Could you check a few things on this model? Use its own coordinates, in mm. A direction names the side the tool comes from. Give positions to 0.01 mm unless a question says otherwise; leave off trailing zeros. Loops run counter-clockwise (first coordinate to the right, second up) from the corner with the lowest first, then second, coordinate; pieces in that order, holes last. Notation, with made-up numbers: (30.5, -17.75) -> (74.5, -17.75) arc R21 cw to (74.5, 1.25) -> close; hole circle Ø7 at (78, 86). An arc over 180 degrees is marked (long way). Write item = value, one per line. Start each with the question number.
1) I need wall thicknesses on probe 1 along Z at (x, y) = (-25, 8.25); probe 2 along Z at (x, y) = (77.5, 13); probe 3 along Y at (x, z) = (-5, -41.5). Which ranges of each line are inside material? Lowest first, please. Write a range as from..to.
2) On a 3-axis mill with a long thin cutter (end or side, diameter ignored), from which of +Z, -Z, +X, -X, +Y, -Y can I reach the whole of each face in a straight line? I mean faces 4 (the face through (-1, 10, 50)), 5 (the face through (-79.73, 56.89, -0.14)), 6 (the face through (-1, 20, 30)). Say none if no direction works.
3) I want a section at A-A (y = 14). Count the separate pieces of the cut face and the enclosed holes in it, and give its area (3 significant figures).
4) I want a section at D-D (y = 43.5). List the corners of the cut face in (x, z) for me.
5) I'm going to push flat-ended pins straight in: pin 1 Ø12 at (x, z) = (-25, -30) entering from +Y; pin 2 Ø24 at (x, z) = (25, -30) entering from +Y; pin 3 Ø1.5 at (x, y) = (74, 27) entering from +Z; pin 4 Ø19.5 at (x, y) = (149, 72) entering from -Z. Where does each tip first touch, or does it pass through?
6) If we mould it in two halves opening along X, with no side actions, what happens to faces 1 (the face through (142.07, 69.13, -0.14)), 2 (the face through (-100, 10, -1)), 3 (the face through (100, 10, -1))? For each: +X half, -X half, draft (parallel to the pull), parting line (faces both ways), or undercut.
7) I want a section at B-B (x = 25). List the corners of the cut face in (y, z) for me, and give its area (3 significant figures).
8) I want a section at C-C (z = -5). List the corners of the cut face in (x, y) for me.
from build123d import *

# Parameters (mm, degrees)
BOSS_EXTRUDE1_DEPTH      = 50
BOSS_EXTRUDE1_DEPTH_BACK = 50
SKETCH1_W                = 200
SKETCH1_H                = 20
BOSS_EXTRUDE2_DEPTH      = 10
BOSS_EXTRUDE2_DEPTH_BACK = 10
HOLE1_D                  = 15
HOLE2_D                  = 15
LPATTERN1_COUNT          = 4
LPATTERN1_PITCH          = 50
MIRROR1_COPY_1_D         = 15
MIRROR1_COPY_2_D         = 15
MIRROR1_COPY_3_D         = 15


with BuildPart() as part:
    # Sketch1 → Boss-Extrude1 (new, two sides: drawn at the far end of the back side and taken through both)
    with BuildSketch(Plane.XY.offset(-BOSS_EXTRUDE1_DEPTH_BACK)):
        with Locations((0, 10)):
            Rectangle(SKETCH1_W, SKETCH1_H)
    extrude(amount=BOSS_EXTRUDE1_DEPTH + BOSS_EXTRUDE1_DEPTH_BACK)

    # Sketch2 → Boss-Extrude2 (add, two sides: drawn at the far end of the back side and taken through both)
    with BuildSketch(Plane.XY.offset(-BOSS_EXTRUDE2_DEPTH_BACK)):
        with BuildLine():
            Line((-141.813369554, 85.613497892), (-15.882414207, 27.348395672))
            ThreePointArc((-15.882414207, 27.348395672), (0, 37.5), (15.882414207, 27.348395672))
            Line((15.882414207, 27.348395672), (142.737764558, 85.630275392))
            ThreePointArc((142.737764558, 85.630275392), (162.01155177, 79.46321114), (157.603646545, 59.712719336))
            Line((157.603646545, 59.712719336), (100.888005584, 20))
            Line((100.888005584, 20), (-100, 20))
            Line((-100, 20), (-156.715640962, 59.712719336))
            ThreePointArc((-156.715640962, 59.712719336), (-161.113566002, 79.480583955), (-141.813369554, 85.613497892))
        make_face()
    extrude(amount=BOSS_EXTRUDE2_DEPTH + BOSS_EXTRUDE2_DEPTH_BACK)

    # Hole1 (through all)
    with Locations(Plane.XY.offset(10)):
        with Locations((-148.111994416, 72), (149, 72)):
            Hole(HOLE1_D / 2)

    # Hole2 (through all)
    with Locations(Plane(origin=(0, 20, 0), x_dir=(1, 0, 0), z_dir=(0, 1, 0))):
        with Locations((75, -30)):
            hole2 = Hole(HOLE2_D / 2)

    # LPattern1: Hole2 ×4
    with Locations(*[(-i * LPATTERN1_PITCH, 0, 0) for i in range(1, LPATTERN1_COUNT)]):
        add(hole2, mode=Mode.SUBTRACT)

    # Mirror1: Hole2 across plane
    add(hole2.mirror(Plane.XY), mode=Mode.SUBTRACT)

    # Mirror1 copy 1 (through all)
    with Locations(Plane(origin=(-50, 20, 0), x_dir=(1, 0, 0), z_dir=(0, 1, 0))):
        with Locations((75, 30)):
            Hole(MIRROR1_COPY_1_D / 2)

    # Mirror1 copy 2 (through all)
    with Locations(Plane(origin=(-100, 20, 0), x_dir=(1, 0, 0), z_dir=(0, 1, 0))):
        with Locations((75, 30)):
            Hole(MIRROR1_COPY_2_D / 2)

    # Mirror1 copy 3 (through all)
    with Locations(Plane(origin=(-150, 20, 0), x_dir=(1, 0, 0), z_dir=(0, 1, 0))):
        with Locations((75, 30)):
            Hole(MIRROR1_COPY_3_D / 2)


solid = part.part
Answer list:
q1.probe_1 = -50..-37.5, -22.5..22.5, 37.5..50
q1.probe_2 = -50..-37.07, -22.93..22.93, 37.07..50
q1.probe_3 = 0..20
q2.face_4 = +Z, +X, -X, +Y, -Y
q2.face_5 = +Z, -Z, +Y
q2.face_6 = +Z, +X, -X, +Y
q3.separate_pieces = 1
q3.enclosed_holes = 8
q3.area = 18,600 mm^2
q4.outline = (-133.56, -10) -> (-50.79, -10) -> (-50.79, 10) -> (-133.56, 10) -> close; (51.04, -10) -> (134.45, -10) -> (134.45, 10) -> (51.04, 10) -> close
q5.pin_1 = through
q5.pin_2 = 20
q5.pin_3 = 10
q5.pin_4 = -10
q6.face_1 = undercut
q6.face_2 = -X half
q6.face_3 = +X half
q7.outline = (0, -50) -> (20, -50) -> (20, -37.5) -> (0, -37.5) -> close; (0, -22.5) -> (20, -22.5) -> (20, -10) -> (31.54, -10) -> (31.54, 10) -> (20, 10) -> (20, 22.5) -> (0, 22.5) -> close; (0, 37.5) -> (20, 37.5) -> (20, 50) -> (0, 50) -> close
q7.area = 1,630 mm^2
q8.outline = (-156.72, 59.71) -> (-100, 20) -> (-100, 0) -> (100, 0) -> (100, 20) -> (100.89, 20) -> (157.6, 59.71) arc R15 ccw to (142.74, 85.63) -> (15.88, 27.35) arc R17.5 ccw to (-15.88, 27.35) -> (-141.81, 85.61) arc R15 ccw to start; hole circle Ø15 at (-148.11, 72); hole circle Ø15 at (149, 72)
